The listing builds one solid part. Answer for the finished solid, in the listing's coordinates (mm). A direction names the side the tool comes from. Give positions to 0.01 mm unless a question says otherwise; leave off trailing zeros. Loops run counter-clockwise (first coordinate to the right, second up) from the corner with the lowest first, then second, coordinate; pieces in that order, holes last.
Item 1: Section A-A, the plane x = 0 is taken. Give the vertices of the cut face in (y, z), and give its area (3 significant figures).
Item 2: The mould has two halves that part along X. Classify faces 5 (the face through (-5.57, -7.96, 3.6)), 6 (the face through (3.859, -7.962, 11.797)), 7 (the face through (9.7, 0, 1.5)), 8 (the face through (0, -10.7, 8)): pulls with the +X half, pulls with the -X half, needs draft (parallel to the pull), parting line crosses it, or undercut.
Item 3: Each of these flat-tipped pins is pushed along its axis until it touches: pin 1 Ø3 at (y, z) = (-8, 7.5) entering from -X; pin 2 Ø2 at (y, z) = (-1.5, 5.5) entering from -X; pin 3 Ø1.2 at (y, z) = (-9, 7) entering from +X; pin 4 Ø4 at (x, y) = (-6, -8.5) entering from +Z. Where does it stop, or does it pass through?
Item 4: Consider line 1 along Y through (x, z) = (0, 1.5); line 2 along Z through (x, y) = (0, -6.85); line 3 along Y through (x, z) = (0, 5.25). Determine where each line is inside the solid, lowest interval first.
Item 5: Section B-B, the plane y = 0 is taken. Give the vertices of the cut face in (x, z), and give its area (3 significant figures).
Item 6: Section D-D, the plane z = 5.5 is taken. Give the vertices of the cut face in (x, y).
Item 7: A tool of negligible diameter and unlimited length cuts with its end or side. For faces 1 (the face through (0, -5.3, 8)), 2 (the face through (11.9, -0.1, 1.5)), 3 (the face through (5, -8, 7)), 4 (the face through (-5, -8, 7)), from which of +Z, -Z, +X, -X, +Y, -Y can it reach the whole face along a straight path? Write none if from no direction.
Item 8: Section C-C, the plane z = 10 is taken. Give the vertices of the cut face in (x, y), and give its area (3 significant figures).
from build123d import *

# Parameters (mm, degrees)
SKETCH_R     = 14.8
SKETCH_R_2   = 3
PAD_DEPTH    = 3
SKETCH002_W  = 10
SKETCH002_H  = 5.4
PAD001_DEPTH = 10
SKETCH003_R  = 1.6
POCKET_DEPTH = 5.4
FILLET_R     = 4
FILLET001_R  = 4
FILLET002_R  = 2
FILLET003_R  = 2


with BuildPart() as part:
    # Sketch → Pad (new body)
    with BuildSketch(Plane.XY):
        Circle(SKETCH_R)
        Circle(SKETCH_R_2, mode=Mode.SUBTRACT)
        with BuildLine():
            ThreePointArc((-9.115018, 3.317595), (-9.772458, 4.727479), (-11.182342, 4.07004))
            ThreePointArc((-11.182342, 4.07004), (-11.9, 0), (-11.182342, -4.07004))
            ThreePointArc((-11.182342, -4.07004), (-9.772458, -4.727479), (-9.115018, -3.317595))
            ThreePointArc((-9.115018, 3.317595), (-9.7, 0), (-9.115018, -3.317595))
        make_face(mode=Mode.SUBTRACT)
        with BuildLine():
            ThreePointArc((11.182342, 4.07004), (9.772458, 4.727479), (9.115018, 3.317595))
            ThreePointArc((9.115018, -3.317595), (9.7, 0), (9.115018, 3.317595))
            ThreePointArc((9.115018, -3.317595), (9.772458, -4.727479), (11.182342, -4.07004))
            ThreePointArc((11.182342, -4.07004), (11.9, 0), (11.182342, 4.07004))
        make_face(mode=Mode.SUBTRACT)
    extrude(amount=PAD_DEPTH)

    # Sketch002 → Pad001 (new body)
    with BuildSketch(Plane.XY.offset(3)):
        with Locations((0, -8)):
            Rectangle(SKETCH002_W, SKETCH002_H)
    extrude(amount=PAD001_DEPTH)

    # Sketch003 → Pocket (cut)
    with BuildSketch(Plane(origin=(0, -5.3, 0), x_dir=(-1, 0, 0), z_dir=(0, 1, 0))):
        with Locations((0, 10)):
            Circle(SKETCH003_R)
    extrude(amount=-POCKET_DEPTH, mode=Mode.SUBTRACT)

    # Fillet
    fillet_edges = [part.edges().sort_by_distance(p)[0] for p in [
        (5, -8, 13),
    ]]
    fillet(fillet_edges, radius=FILLET_R)

    # Fillet001
    fillet001_edges = [part.edges().sort_by_distance(p)[0] for p in [
        (-5, -8, 13),
    ]]
    fillet(fillet001_edges, radius=FILLET001_R)

    # Fillet002
    fillet002_edges = [part.edges().sort_by_distance(p)[0] for p in [
        (5, -8, 3),
    ]]
    fillet(fillet002_edges, radius=FILLET002_R)

    # Fillet003
    fillet003_edges = [part.edges().sort_by_distance(p)[0] for p in [
        (-5, -8, 3),
    ]]
    fillet(fillet003_edges, radius=FILLET003_R)


solid = part.part
Worked answers:
1. outline: (-14.8, 0) - (-3, 0) - (-3, 3) - (-5.3, 3) - (-5.3, 8.4) - (-10.7, 8.4) - (-10.7, 3) - (-14.8, 3) - close; (-10.7, 11.6) - (-5.3, 11.6) - (-5.3, 13) - (-10.7, 13) - close; (3, 0) - (14.8, 0) - (14.8, 3) - (3, 3) - close
1. area: 108 mm2
2. face 5: pulls with the -X half
2. face 6: pulls with the +X half
2. face 7: undercut
2. face 8: needs draft
3. pin 1: stops at x = -5
3. pin 2: passes through
3. pin 3: stops at x = 5
3. pin 4: stops at z = 11.65
4. line 1: y = -14.8 to -3, 3 to 14.8
4. line 2: z = 0 to 8.4, 11.6 to 13
4. line 3: y = -10.7 to -5.3
5. outline: (-14.8, 0) - (-11.9, 0) - (-11.9, 3) - (-14.8, 3) - close; (-9.7, 0) - (-3, 0) - (-3, 3) - (-9.7, 3) - close; (3, 0) - (9.7, 0) - (9.7, 3) - (3, 3) - close; (11.9, 0) - (14.8, 0) - (14.8, 3) - (11.9, 3) - close
5. area: 57.6 mm2
6. outline: (-5, -10.7) - (5, -10.7) - (5, -5.3) - (-5, -5.3) - close
7. face 1: +Z, +X, -X, +Y
7. face 2: +Z, -Z
7. face 3: +Z, +X, +Y, -Y
7. face 4: +Z, -X, +Y, -Y
8. outline: (-4.87, -10.7) - (-1.6, -10.7) - (-1.6, -5.3) - (-4.87, -5.3) - close; (1.6, -10.7) - (4.87, -10.7) - (4.87, -5.3) - (1.6, -5.3) - close
8. area: 35.3 mm2
